Input: part model. Units: mm. Frame: model coordinates. A direction names the side the tool comes from. Coordinates: 2 decimals unless noted, no trailing zeros. Order: outer loops, then holes, each group sorted by start corner. A loop starts at its lowest first (then second) coordinate and runs counter-clockwise, first axis right, second up. Notation, with made-up numbers: M -14,82 L -10,82 A26 cw -10,99 Z; hole C 38.5,5 d9. An arc over 180 degrees is marked long. Answer in a Markdown table with one row per item.
from build123d import *

# Parameters (mm, degrees)
F1_DEPTH = 14
F2_W     = 46
F2_H     = 24
F3_DEPTH = 55
F4_R     = 0.997642
F5_DEPTH = 2.5
F6_W     = 67
F6_H     = 67
F7_DEPTH = 5
F8_R     = 3
F9_DEPTH = 25


with BuildPart() as f1:
    # F0 (on Top) → F1 (new body, symmetric)
    with BuildSketch(Plane.XY):
        with BuildLine():
            Line((43, 42), (-5, 42))
            Line((-5, 42), (-5, -6))
            ThreePointArc((-5, -6), (28.941125, 8.058875), (43, 42))
        make_face()
    extrude(amount=F1_DEPTH, both=True)

    # F2 (on face) → F3 (cut)
    with BuildSketch(Plane(origin=(-5, 0, 0), x_dir=(0, -1, 0), z_dir=(-1, 0, 0))):
        with Locations((-17, 0)):
            Rectangle(F2_W, F2_H)
    extrude(amount=-F3_DEPTH, mode=Mode.SUBTRACT)

    # F4 (on face) → F5 (join)
    with BuildSketch(Plane.XY.offset(14)):
        Circle(F4_R)
    extrude(amount=-F5_DEPTH)

    # F6 (on face) → F7 (join)
    with BuildSketch(Plane(origin=(0, 42, 0), x_dir=(-1, 0, 0), z_dir=(0, 1, 0))):
        with Locations((-24.5, 0)):
            Rectangle(F6_W, F6_H)
    extrude(amount=F7_DEPTH)

    # F8 (on face) → F9 (cut)
    with BuildSketch(Plane(origin=(0, 47, 0), x_dir=(-1, 0, 0), z_dir=(0, 1, 0))):
        with Locations((-47, 22.5)):
            Circle(F8_R)
        with Locations((-3, 22.5)):
            Circle(F8_R)
        with Locations((-47, -21.5)):
            Circle(F8_R)
        with Locations((-3, -21.5)):
            Circle(F8_R)
    extrude(amount=-F9_DEPTH, mode=Mode.SUBTRACT)


solid = f1.part
1) Cut plane D-D, the plane z = 1. Output: boundary loops of the cut face in (x, y), and give its area (3 significant figures).
Resolved:
| item | result |
|---|---|
| outline | M -9,42 L -5,42 L -5,40 L 42.96,40 A48 ccw 43,42 L 58,42 L 58,47 L -9,47 Z |
| area | 431 mm2 |
2) Material intervals for probe 1 along Z at (x, y) = (47, 44.35); probe 2 along Z at (x, y) = (23.5, 14); probe 3 along Y at (x, z) = (31, 21), sorted ascending.
Resolved:
| item | result |
|---|---|
| probe 1 | z = -33.5 to -24.5, -18.5 to 19.5, 25.5 to 33.5 |
| probe 2 | z = -14 to -12, 12 to 14 |
| probe 3 | y = 42 to 47 |
3) Contact query for flat-ended pins moving along their axis: pin 1 (23 mm diameter, centred on x = 21, y = 27.5, fed in from -Z); pin 2 (14 mm diameter, centred on x = 27.5, y = 11.5, fed in from +Z); pin 3 (5.5 mm diameter, centred on x = 3, z = 22.5, fed in from -Y); pin 4 (12 mm diameter, centred on x = 29, z = 1, fed in from -Y). Output: stop coordinate, or through.
Resolved:
| item | result |
|---|---|
| pin 1 | stops at z = -14 |
| pin 2 | stops at z = 14 |
| pin 3 | passes through |
| pin 4 | stops at y = 40 |
4) Cut plane B-B, the plane z = -21.5. Output: boundary loops of the cut face in (x, y).
Resolved:
| item | result |
|---|---|
| outline | M -9,42 L 0,42 L 0,47 L -9,47 Z; M 6,42 L 44,42 L 44,47 L 6,47 Z; M 50,42 L 58,42 L 58,47 L 50,47 Z |
5) Cut plane C-C, the plane y = 14.5. Output: boundary loops of the cut face in (x, z).
Resolved:
| item | result |
|---|---|
| outline | M -5,-14 L 34.34,-14 L 34.34,-12 L -5,-12 Z; M -5,12 L 34.34,12 L 34.34,14 L -5,14 Z |
6) Reachability of faces 4 (the face through (13, 24, 14)), 5 (the face through (0, 0, 11.5)), 6 (the face through (13, 24, -14)), 7 (the face through (25, 47, 0)) from +Z, -Z, +X, -X, +Y, -Y: full face, straight path, thin tool, end or side. Return the list, or none.
Resolved:
| item | result |
|---|---|
| face 4 | +Z, +X, -X, -Y |
| face 5 | +X, -X, -Y |
| face 6 | -Z, +X, -X, -Y |
| face 7 | +Z, -Z, +X, -X, +Y |
7) Mould query, pull axis Y, two halves, no side actions, for faces 1 (the face through (32.54, 12.09, -12.38)), 2 (the face through (-0.79, -0.61, 11.75)), 3 (the face through (25, 44, 33.5)). Classes: +Y half, -Y half, draft (parallel to the pull), parting line (faces both ways), or undercut.
Resolved:
| item | result |
|---|---|
| face 1 | -Y half |
| face 2 | undercut |
| face 3 | draft |
8) Cut plane A-A, the plane x = 47. Output: boundary loops of the cut face in (y, z), and give its area (3 significant figures).
Resolved:
| item | result |
|---|---|
| outline | M 42,-33.5 L 47,-33.5 L 47,-24.5 L 42,-24.5 Z; M 42,-18.5 L 47,-18.5 L 47,19.5 L 42,19.5 Z; M 42,25.5 L 47,25.5 L 47,33.5 L 42,33.5 Z |
| area | 275 mm2 |
